from build123d import *


with BuildPart() as part:
    # Sketch1 → Revolve1 (revolve)
    with BuildSketch(Plane.XY, mode=Mode.PRIVATE) as revolve1_sk:
        with BuildLine():
            Line((28.176458362, 0), (32.4, 0))
            ThreePointArc((32.4, 0), (34.167766953, 0.732233047), (34.9, 2.5))
            Line((34.9, 2.5), (34.9, 184))
            add(Edge.make_bspline(
                [(34.9, 184), (34.9, 186.989827139), (31.915630123, 192.216128506), (25.82490647, 195.027230742), (22, 197.912231806), (22, 200)],
                knots=[0, 0, 0, 0, 0.423782802, 0.726128109, 1, 1, 1, 1], degree=3))
            Line((22, 200), (22, 207.75))
            ThreePointArc((22, 207.75), (21.707106781, 208.457106781), (21, 208.75))
            Line((21, 208.75), (19.968095661, 208.75))
            ThreePointArc((19.968095661, 208.75), (18.587521001, 209.302929301), (17.970306523, 210.655986393))
            Line((17.970306523, 210.655986393), (17.06, 230))
            Line((17.06, 230), (0, 230))
            Line((0, 230), (0, 1))
            Line((0, 1), (24.371019058, 1))
            ThreePointArc((24.371019058, 1), (24.891963591, 0.954423259), (25.397079488, 0.819077862))
            Line((25.397079488, 0.819077862), (27.150397932, 0.180922138))
            ThreePointArc((27.150397932, 0.180922138), (27.655513829, 0.045576741), (28.176458362, 0))
        make_face()
    revolve(revolve1_sk.sketch.rotate(Axis((0, 0, 0), (0, 1, 0)), 90), axis=Axis((0, 0, 0), (0, 1, 0)))


solid = part.part
Source: CAD feature listing. Evaluate the final solid. Frame: model axes, mm. A direction names the side the tool comes from. Give positions to 0.01 mm unless a question says otherwise; leave off trailing zeros. Order: outer loops, then holes, each group sorted by start corner. A loop starts at its lowest first (then second) coordinate and runs counter-clockwise, first axis right, second up. Notation, with made-up numbers: (-14.5, 30.25) -> (35.5, 30.25) arc R16 cw to (35.5, 38.25) -> close; hole circle Ø7 at (9, -24.5). An arc over 180 degrees is marked (long way). Write item = value, one per line.
Q1. Cut plane A-A, the plane y = 180. Output: boundary loops of the cut face in (x, z).
Data:
outline = circle Ø69.8 at (0, 0)
Q2. Pull-direction query (X, two-part tool) for faces 1 (the face through (0, 230, 0)), 2 (the face through (0, 1, 0)), 3 (the face through (-17.36, 220.46, 2.28)); classes: released by +X, released by -X, zero draft, split by the parting line, or undercut.
Data:
face_1 = zero draft
face_2 = undercut
face_3 = split by the parting line
Q3. Set-up query: faces 4 (the face through (-27, 0, -10)), 5 (the face through (21.477, 203.929, 4.769)). Return all of +Z, -Z, +X, -X, +Y, -Y with unobstructed straight access to the full face (end or side cutting, diameter ignored); none if empty.
Data:
face_4 = +Z, -Z, +X, -X, -Y
face_5 = +Y
Q4. Material intervals for line 1 (X direction, y = 162, z = 1.5); line 2 (Y direction, x = -8, z = -18); line 3 (Y direction, x = -7, z = -10), sorted ascending. Write a range as from..to.
Data:
line_1 = -34.87..34.87
line_2 = 1..208.77
line_3 = 1..230
Q5. Pin query (flat end, axial travel): pin 1 (10 mm diameter, centred on y = 133.5, z = -5.5, fed in from +X); pin 2 (5 mm diameter, centred on x = 4, z = -21, fed in from +Y); pin 3 (1 mm diameter, centred on x = -7, y = 95, fed in from -Z). Return the tip coordinate at first contact, or that it passes through.
Data:
pin_1 = 34.9
pin_2 = 209.07
pin_3 = -34.29
